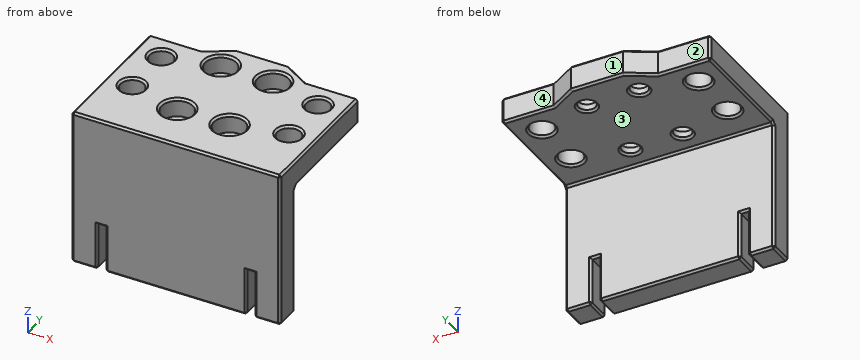
```python
from build123d import *

# Parameters (mm, degrees)
SKETCH1_W           = 40
SKETCH1_H           = 27
BOSS_EXTRUDE1_DEPTH = 5
SKETCH2_W           = 40
SKETCH2_H           = 5
BOSS_EXTRUDE2_DEPTH = 25
SKETCH3_R           = 1.65
CUT_EXTRUDE1_DEPTH  = 15
BOSS_EXTRUDE3_DEPTH = 5
SKETCH5_R           = 3
CUT_EXTRUDE2_DEPTH  = 3.5
SKETCH6_W           = 1.5
SKETCH6_H           = 9
CUT_EXTRUDE3_DEPTH  = 5
SKETCH7_R           = 2.25
CUT_EXTRUDE4_DEPTH  = 5
CHAMFER1_SIZE       = 0.4


with BuildPart() as part:
    # Sketch1 → Boss-Extrude1 (new body)
    with BuildSketch(Plane.XY):
        Rectangle(SKETCH1_W, SKETCH1_H)
    extrude(amount=BOSS_EXTRUDE1_DEPTH)

    # Sketch2 → Boss-Extrude2 (add)
    with BuildSketch(Plane(origin=(0, 0, 0), x_dir=(-1, 0, 0), z_dir=(0, 0, -1))):
        with Locations((0, -11)):
            Rectangle(SKETCH2_W, SKETCH2_H)
    extrude(amount=BOSS_EXTRUDE2_DEPTH)

    # Sketch3 → Cut-Extrude1 (cut)
    with BuildSketch(Plane.XY.offset(5)):
        with Locations((-5, 11)):
            Circle(SKETCH3_R)
        with Locations((5, 11)):
            Circle(SKETCH3_R)
        with Locations((5, -4)):
            Circle(SKETCH3_R)
        with Locations((-5, -4)):
            Circle(SKETCH3_R)
    extrude(amount=-CUT_EXTRUDE1_DEPTH, mode=Mode.SUBTRACT)

    # Sketch4 → Boss-Extrude3 (add)
    with BuildSketch(Plane.XY.offset(5)):
        Polygon((-10, 13.5), (-5, 16.5), (5, 16.5), (10, 13.5), align=None)
    extrude(amount=-BOSS_EXTRUDE3_DEPTH)

    # Sketch5 → Cut-Extrude2 (cut)
    with BuildSketch(Plane.XY.offset(5)):
        with Locations((-5, 11)):
            Circle(SKETCH5_R)
        with Locations((5, 11)):
            Circle(SKETCH5_R)
        with Locations((5, -4)):
            Circle(SKETCH5_R)
        with Locations((-5, -4)):
            Circle(SKETCH5_R)
    extrude(amount=-CUT_EXTRUDE2_DEPTH, mode=Mode.SUBTRACT)

    # Sketch6 → Cut-Extrude3 (cut)
    with BuildSketch(Plane(origin=(0, -8.5, 0), x_dir=(1, 0, 0), z_dir=(0, 1, 0))):
        with Locations((-14.25, 20.5)):
            Rectangle(SKETCH6_W, SKETCH6_H)
        with Locations((14.25, 20.5)):
            Rectangle(SKETCH6_W, SKETCH6_H)
    extrude(amount=-CUT_EXTRUDE3_DEPTH, mode=Mode.SUBTRACT)

    # Sketch7 → Cut-Extrude4 (cut)
    with BuildSketch(Plane.XY.offset(5)):
        with Locations((-15, 8.5)):
            Circle(SKETCH7_R)
        with Locations((15, 8.5)):
            Circle(SKETCH7_R)
        with Locations((15, -1.5)):
            Circle(SKETCH7_R)
        with Locations((-15, -1.5)):
            Circle(SKETCH7_R)
    extrude(amount=-CUT_EXTRUDE4_DEPTH, mode=Mode.SUBTRACT)

    # Chamfer1
    chamfer1_edges = [part.edges().sort_by_distance(p)[0] for p in [
        (-15, -13.5, -20.5),
        (-15, -11, -25),
        (-13.5, -13.5, -20.5),
        (-13.5, -11, -25),
        (-14.25, -13.5, -16),
        (-15, -8.5, -20.5),
        (-14.25, -8.5, -16),
        (-13.5, -8.5, -20.5),
        (13.5, -13.5, -20.5),
        (13.5, -11, -25),
        (15, -13.5, -20.5),
        (15, -11, -25),
        (14.25, -13.5, -16),
        (13.5, -8.5, -20.5),
        (14.25, -8.5, -16),
        (15, -8.5, -20.5),
        (-17.25, -1.5, 0),
        (-17.25, -1.5, 5),
        (-20, 0, 5),
        (12.75, -1.5, 0),
        (12.75, -1.5, 5),
        (12.75, 8.5, 0),
        (12.75, 8.5, 5),
        (-17.25, 8.5, 0),
        (-17.25, 8.5, 5),
        (20, 2.5, 0),
        (20, -8.5, -12.5),
        (0, -8.5, 0),
        (0, -13.5, 5),
        (-20, -8.5, -12.5),
        (20, -11, -25),
        (17.5, -13.5, -25),
        (-20, -11, -25),
        (-17.5, -8.5, -25),
        (-6.65, -4, 0),
        (3.35, -4, 0),
        (3.35, 11, 0),
        (-6.65, 11, 0),
        (-15, 13.5, 0),
        (-15, 13.5, 5),
        (20, 0, 5),
        (-7.5, 15, 0),
        (0, 16.5, 0),
        (7.5, 15, 0),
        (7.5, 15, 5),
        (0, 16.5, 5),
        (-7.5, 15, 5),
        (-20, 2.5, 0),
        (15, 13.5, 0),
        (-8, -4, 5),
        (2, -4, 5),
        (2, 11, 5),
        (-8, 11, 5),
        (20, -13.5, -10),
        (-20, -13.5, -10),
        (-20, 13.5, 2.5),
        (20, 13.5, 2.5),
        (0, -13.5, -25),
        (15, 13.5, 5),
        (-17.5, -13.5, -25),
        (0, -8.5, -25),
        (17.5, -8.5, -25),
    ]]
    chamfer(chamfer1_edges, length=CHAMFER1_SIZE)


solid = part.part
```
Part model, mm, in its own coordinate system. Face numbers are marked on the shaded views. A direction names the side the tool comes from. Round coordinates to 2 decimals unless told otherwise and drop trailing zeros. Write each loop counter-clockwise with the first axis right and the second up, starting at its lowest first coordinate (ties: lowest second). Pieces come first, ordered by that corner, then holes. Notation, with made-up numbers: M 11.25,84 L 49.25,84 A31 cw 49.25,115 Z; hole C 79,33.25 d5. An arc over 180 degrees is marked long. One line per question, with ' | ' between items.
(1) 3-axis set-ups, long thin cutter, end or side, ignore diameter. For the marked faces 1, 2, 3 and 4: which of +Z, -Z, +X, -X, +Y, -Y reach the whole face in a straight line?
Answer key:
face 1: +Z, -Z, +X, -X, +Y | face 2: +Z, -Z, -X, +Y | face 3: -Z, +X, -X, +Y | face 4: +Z, -Z, +X, +Y
(2) Pin check, flat tips, straight feed: pin 1 (1.2 mm diameter, centred on x = -14, y = -11, fed in from -Z); pin 2 (1.5 mm diameter, centred on x = -10, y = -2, fed in from -Z); pin 3 (3 mm diameter, centred on x = 3.5, y = -3.5, fed in from +Z); pin 4 (2.5 mm diameter, centred on x = 15, y = -1.5, fed in from +Z). Stop position of each tip, or through.
Answer key:
pin 1: stops at z = -24.7 | pin 2: stops at z = 0 | pin 3: stops at z = 4.68 | pin 4: passes through
(3) Saw through at C-C on y = 3.5. Write the cut outline in (x, z).
Answer key:
outline: M -20,0.4 L -19.6,0 L 19.6,0 L 20,0.4 L 20,4.6 L 19.6,5 L -19.6,5 L -20,4.6 Z
(4) Probe line 1 along Y through (x, z) = (-5, 3); line 2 along Y through (x, z) = (-15, 1); line 3 along Z through (x, y) = (5.5, 2.75). List the from-to ranges inside material, lowest first.
Answer key:
line 1: y = -13.5 to -7, -1 to 8, 14 to 16.5 | line 2: y = -13.5 to -3.75, 0.75 to 6.25, 10.75 to 13.5 | line 3: z = 0 to 5
(5) Saw through at A-A on z = -16.5. Write the cut outline in (x, y), then the cut area to 3 significant figures.
Answer key:
outline: M -20,-13.1 L -19.6,-13.5 L -15.4,-13.5 L -15,-13.1 L -15,-8.9 L -15.4,-8.5 L -19.6,-8.5 L -20,-8.9 Z; M -13.5,-13.1 L -13.1,-13.5 L 13.1,-13.5 L 13.5,-13.1 L 13.5,-8.9 L 13.1,-8.5 L -13.1,-8.5 L -13.5,-8.9 Z; M 15,-13.1 L 15.4,-13.5 L 19.6,-13.5 L 20,-13.1 L 20,-8.9 L 19.6,-8.5 L 15.4,-8.5 L 15,-8.9 Z | area: 184 mm^2
(6) Saw through at B-B on z = -13. Write the cut outline in (x, y), then the cut area to 3 significant figures.
Answer key:
outline: M -20,-13.1 L -19.6,-13.5 L 19.6,-13.5 L 20,-13.1 L 20,-8.9 L 19.6,-8.5 L -19.6,-8.5 L -20,-8.9 Z | area: 200 mm^2
